Part model, mm, in its own coordinate system. Round coordinates to 2 decimals unless told otherwise and drop trailing zeros. Write each loop counter-clockwise with the first axis right and the second up, starting at its lowest first coordinate (ties: lowest second). Pieces come first, ordered by that corner, then holes.
1) Drill centre lines: L1, parallel to X at y = 0.95, z = 8; L2, parallel to Z at x = -1.25, y = 2.3; L3, parallel to Z at x = -7.75, y = 1.1. Where is each one in solid material? Low to high.
2) Flat gauge pin, fed straight in: pin 1 (4 mm diameter, centred on x = -7, z = 15, fed in from +Y). Where does the tip first touch, or does it go through?
3) Saw through at A-A on z = 15. Write the cut outline in (x, y), and give its area (3 significant figures).
4) Saw through at C-C on y = 1.1. Write the cut outline in (x, z), and give its area (3 significant figures).
5) Saw through at D-D on z = 8. Write the cut outline in (x, y), and give its area (3 significant figures).
6) Saw through at B-B on x = 0. Write the cut outline in (y, z).
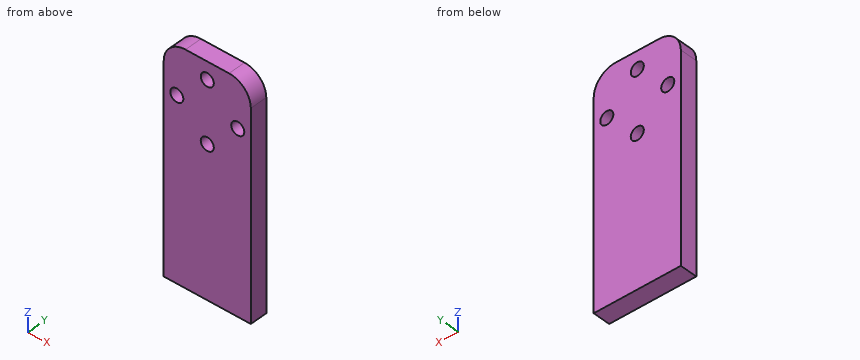
```python
from build123d import *

# Parameters (mm, degrees)
SKETCH1_W           = 20
SKETCH1_H           = 52
SKETCH1_R           = 1.5
BOSS_EXTRUDE1_DEPTH = 4
FILLET1_R           = 5


with BuildPart() as part:
    # Sketch1 → Boss-Extrude1 (new body)
    with BuildSketch(Plane(origin=(0, 0, 0), x_dir=(1, 0, 0), z_dir=(0, 1, 0))):
        Rectangle(SKETCH1_W, SKETCH1_H)
        with Locations(Location((0, -22, 0), (0, 0, 270))):
            Circle(SKETCH1_R, mode=Mode.SUBTRACT)
        with Locations(Location((0, -8, 0), (0, 0, 270))):
            Circle(SKETCH1_R, mode=Mode.SUBTRACT)
        with Locations(Location((7, -15, 0), (0, 0, 270))):
            Circle(SKETCH1_R, mode=Mode.SUBTRACT)
        with Locations(Location((-7, -15, 0), (0, 0, 270))):
            Circle(SKETCH1_R, mode=Mode.SUBTRACT)
    extrude(amount=BOSS_EXTRUDE1_DEPTH)

    # Fillet1
    fillet1_edges = [part.edges().sort_by_distance(p)[0] for p in [
        (10, 2, 26),
        (-10, 2, 26),
    ]]
    fillet(fillet1_edges, radius=FILLET1_R)


solid = part.part
```
Completed:
1. L1: x = -10 to -1.5, 1.5 to 10
1. L2: z = -26 to 7.17, 8.83 to 21.17, 22.83 to 26
1. L3: z = -26 to 13.7, 16.3 to 25.18
2. pin 1: stops at y = 4
3. outline: (-10, 0) - (-8.5, 0) - (-8.5, 4) - (-10, 4) - close; (-5.5, 0) - (5.5, 0) - (5.5, 4) - (-5.5, 4) - close; (8.5, 0) - (10, 0) - (10, 4) - (8.5, 4) - close
3. area: 56.0 mm2
4. outline: (-10, -26) - (10, -26) - (10, 21) arc R5 ccw to (5, 26) - (-5, 26) arc R5 ccw to (-10, 21) - close; hole circle Ø3 at (-7, 15); hole circle Ø3 at (0, 8); hole circle Ø3 at (0, 22); hole circle Ø3 at (7, 15)
4. area: 1,000 mm2
5. outline: (-10, 0) - (-1.5, 0) - (-1.5, 4) - (-10, 4) - close; (1.5, 0) - (10, 0) - (10, 4) - (1.5, 4) - close
5. area: 68.0 mm2
6. outline: (0, -26) - (4, -26) - (4, 6.5) - (0, 6.5) - close; (0, 9.5) - (4, 9.5) - (4, 20.5) - (0, 20.5) - close; (0, 23.5) - (4, 23.5) - (4, 26) - (0, 26) - close
